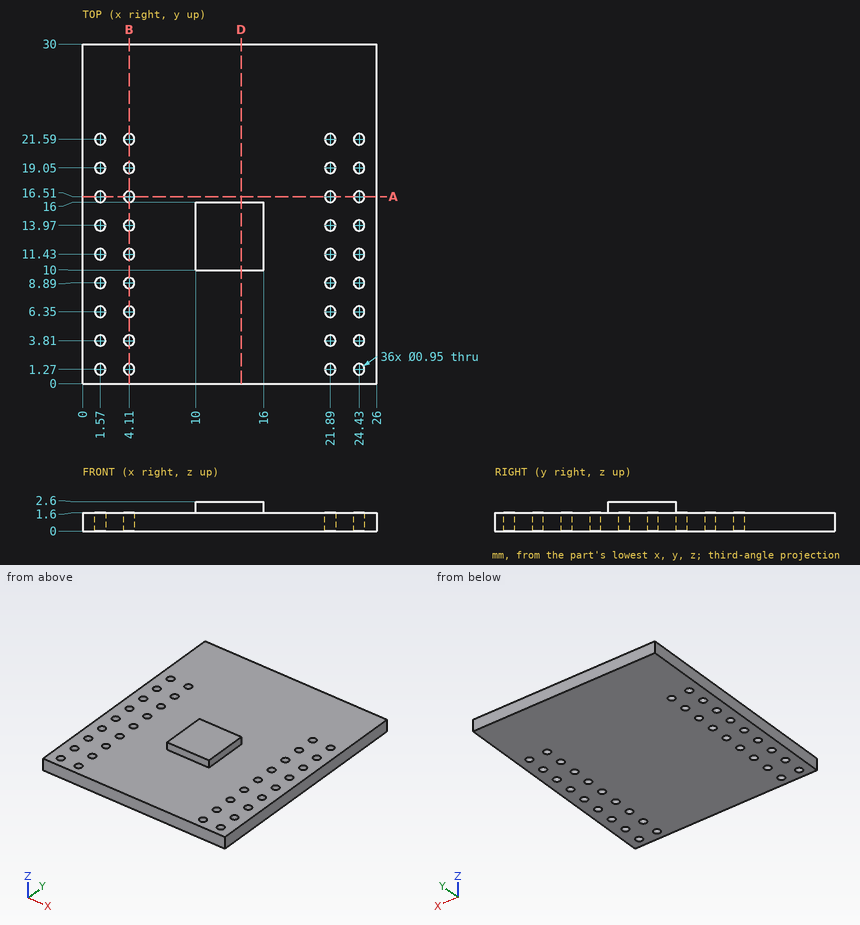
Could you check a few things on this drawing? It's one solid part, dimensions in mm from its lowest x, y, z. Coordinates: 2 decimals unless noted, no trailing zeros. Loops run counter-clockwise (first coordinate to the right, second up) from the corner with the lowest first, then second, coordinate; pieces in that order, holes last.
1. For P1, Ø0.5, axis at x = 11.5, z = 2, coming from the -Y side, with a flat end and sliding along its axis, tell me the tip position at first contact or that it passes through.
2. Imagine slicing it at D-D (x = 14). Please give me the cut outline in (y, z), and give its area (3 significant figures).
3. Imagine slicing it at A-A (y = 16.51). Please give me the cut outline in (x, z) (3 decimals).
4. Imagine slicing it at B-B (x = 4.11). Give the number of separate pieces and of enclosed holes in the cut face, and give its area (3 significant figures).
5. I need wall thicknesses on L1, parallel to X at y = 13.97, z = 1.05 (3 decimals); L2, parallel to Z at x = 14.5, y = 28.5. Which ranges of each line are inside material? Lowest first, please.
Computed values:
1. P1: stops at y = 10
2. outline: (0, 0) - (30, 0) - (30, 1.6) - (16, 1.6) - (16, 2.6) - (10, 2.6) - (10, 1.6) - (0, 1.6) - close
2. area: 54.0 mm2
3. outline: (0, 0) - (1.095, 0) - (1.095, 1.6) - (0, 1.6) - close; (2.045, 0) - (3.635, 0) - (3.635, 1.6) - (2.045, 1.6) - close; (4.585, 0) - (21.415, 0) - (21.415, 1.6) - (4.585, 1.6) - close; (22.365, 0) - (23.955, 0) - (23.955, 1.6) - (22.365, 1.6) - close; (24.905, 0) - (26, 0) - (26, 1.6) - (24.905, 1.6) - close
4. separate pieces: 10
4. enclosed holes: 0
4. area: 34.3 mm2
5. L1: x = 0 to 1.095, 2.045 to 3.635, 4.585 to 21.415, 22.365 to 23.955, 24.905 to 26
5. L2: z = 0 to 1.6
